The model under review builds one solid part; all positions refer to its coordinate system, in mm. Face numbers are marked on the shaded views. A direction names the side the tool comes from. Give positions to 0.01 mm unless a question says otherwise; leave off trailing zeros. Order: outer loops, then holes, each group sorted by start corner. A loop starts at its lowest first (then second) coordinate and runs counter-clockwise, first axis right, second up. Notation, with made-up numbers: (-32, 42.25) - (1, 42.25) arc R29 ccw to (1, 79.25) - close; hole circle Ø8 at (29, -7.75). An arc over 180 degrees is marked (long way). Use CSV: the item, a comma, the result in double quotes. Start each with the question number.
1. Draft analysis for pull direction Z (two halves, no side actions). For the marked faces 3, 4 and 5, state which applies: released by +Z, released by -Z, zero draft, split by the parting line, or undercut.
2. Take a section at A-A, the plane y = 0. State the section outline as (x, z) points.
3. Take a section at D-D, the plane y = 11.5. State the section outline as (x, z) points.
4. Take a section at C-C, the plane z = 4.25. State the section outline as (x, y) points, then the cut area to 3 significant figures.
5. Machinability: for the marked faces 1 and 2, which of the approach directions +Z, -Z, +X, -X, +Y, -Y give a long, thin tool a straight path to every point of the face, cutting with its end or side? Answer none if there is none.
6. To check wall thickness, follow line 1 (Y direction, x = 0, z = 1.75); line 2 (Z direction, x = -11, y = 10.5); line 3 (X direction, y = -1, z = -3.25). State the ranges of each line that lie inside material, in increasing order. Write a range as [from, to].
7. For pin 1 (6 mm diameter, centred on y = -7.5, z = 4, fed in from +X); pin 2 (2 mm diameter, centred on y = 8.5, z = -1.5, fed in from +X); pin 3 (1 mm diameter, centred on y = 10.5, z = 1.5, fed in from +X); pin 4 (3.5 mm diameter, centred on x = 0, y = 0, fed in from -Z), all flat-tipped, find the tip position at first contact; note any pin that passes through.
```python
from build123d import *

# Parameters (mm, degrees)
SKETCH1_R           = 12.7
BOSS_EXTRUDE1_DEPTH = 3.048
SKETCH2_R           = 15.24
BOSS_EXTRUDE2_DEPTH = 3
SKETCH3_R           = 3
CUT_EXTRUDE1_DEPTH  = 25.606


with BuildPart() as part:
    # Sketch1 → Boss-Extrude1 (new body, symmetric)
    with BuildSketch(Plane.XY):
        Circle(SKETCH1_R)
    extrude(amount=BOSS_EXTRUDE1_DEPTH, both=True)

    # Sketch2 → Boss-Extrude2 (add)
    with BuildSketch(Plane.XY.offset(3.048)):
        Circle(SKETCH2_R)
    boss_extrude2 = extrude(amount=BOSS_EXTRUDE2_DEPTH)

    # Mirror1: Boss-Extrude2 across plane
    add(boss_extrude2.mirror(Plane.XY))

    # Sketch3 → Cut-Extrude1 (cut)
    with BuildSketch(Plane.XY.offset(6.048)):
        Circle(SKETCH3_R)
    extrude(amount=-CUT_EXTRUDE1_DEPTH, mode=Mode.SUBTRACT)


solid = part.part
```
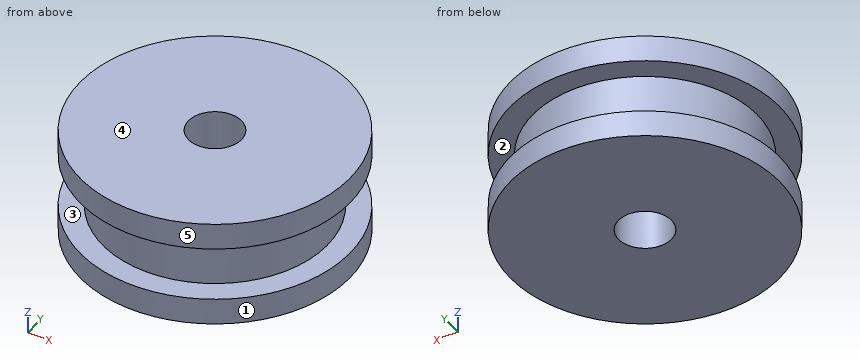
Determined:
1,face 3,"undercut"
1,face 4,"released by +Z"
1,face 5,"zero draft"
2,outline,"(-15.24, -6.05) - (-3, -6.05) - (-3, 6.05) - (-15.24, 6.05) - (-15.24, 3.05) - (-12.7, 3.05) - (-12.7, -3.05) - (-15.24, -3.05) - close; (3, -6.05) - (15.24, -6.05) - (15.24, -3.05) - (12.7, -3.05) - (12.7, 3.05) - (15.24, 3.05) - (15.24, 6.05) - (3, 6.05) - close"
3,outline,"(-10, -6.05) - (10, -6.05) - (10, -3.05) - (5.39, -3.05) - (5.39, 3.05) - (10, 3.05) - (10, 6.05) - (-10, 6.05) - (-10, 3.05) - (-5.39, 3.05) - (-5.39, -3.05) - (-10, -3.05) - close"
4,outline,"circle Ø30.48 at (0, 0); hole circle Ø6 at (0, 0)"
4,area,"701 mm²"
5,face 1,"+Z, -Z"
5,face 2,"none"
6,line 1,"y = [-12.7, -3], [3, 12.7]"
6,line 2,"z = [-6.05, -3.05], [3.05, 6.05]"
6,line 3,"x = [-15.21, -2.83], [2.83, 15.21]"
7,pin 1,"stops at x = 14.56"
7,pin 2,"stops at x = 10.25"
7,pin 3,"stops at x = 7.83"
7,pin 4,"passes through"
